```python
from build123d import *

# Parameters (mm, degrees)
F0_W      = 5.5
F0_H      = 9.5
F1_DEPTH  = 32
F2_SIZE   = 1
F3_R      = 1.5
F4_DEPTH  = 5.5
F5_W      = 1.5
F5_H      = 8
F6_DEPTH  = 9.5
F8_DEPTH  = 1
F10_DEPTH = 1
F11_R     = 1.5
F12_DEPTH = 9.5


with BuildPart() as f1:
    # F0 (on Top) → F1 (new body)
    with BuildSketch(Plane.XY):
        with Locations((2.75, 4.75)):
            Rectangle(F0_W, F0_H)
    extrude(amount=F1_DEPTH)

    # F2
    f2_edges = [f1.edges().sort_by_distance(p)[0] for p in [
        (2.75, 0, 32),
        (2.75, 9.5, 32),
    ]]
    chamfer(f2_edges, length=F2_SIZE)

    # F3 (on face) → F4 (cut, through all)
    with BuildSketch(Plane.YZ.offset(5.5)):
        with Locations((4.75, 3)):
            Circle(F3_R)
    extrude(amount=-F4_DEPTH, mode=Mode.SUBTRACT)

    # F5 (on face) → F6 (cut, through all)
    with BuildSketch(Plane(origin=(0, 9.5, 0), x_dir=(-1, 0, 0), z_dir=(0, 1, 0))):
        with Locations((-2.75, 4)):
            Rectangle(F5_W, F5_H)
    extrude(amount=-F6_DEPTH, mode=Mode.SUBTRACT)

    # F7 (on face) → F8 (cut)
    with BuildSketch(Plane.YZ.offset(5.5)):
        Polygon((9.5, 17), (0, 29), (0, 28), (9.5, 16), align=None)
    extrude(amount=-F8_DEPTH, mode=Mode.SUBTRACT)

    # F9 (on face) → F10 (cut)
    with BuildSketch(Plane(origin=(0, 0, 0), x_dir=(0, -1, 0), z_dir=(-1, 0, 0))):
        Polygon((0, 28), (0, 29), (-9.5, 17), (-9.5, 16), align=None)
    extrude(amount=-F10_DEPTH, mode=Mode.SUBTRACT)

    # F11 (on face) → F12 (cut, through all)
    with BuildSketch(Plane.XZ):
        with Locations((2.75, 21.25)):
            Circle(F11_R)
    extrude(amount=-F12_DEPTH, mode=Mode.SUBTRACT)


solid = f1.part
```
For this review, take the finished solid that the model builds, in its own axes (mm). A direction names the side the tool comes from. Round coordinates to 2 decimals unless told otherwise and drop trailing zeros. Write each loop counter-clockwise with the first axis right and the second up, starting at its lowest first coordinate (ties: lowest second). Pieces come first, ordered by that corner, then holes. Notation, with made-up numbers: (-25.5, -19) - (32.5, -19) arc R19 cw to (32.5, -5) - close; hole circle Ø9 at (10, 58.25). An arc over 180 degrees is marked (long way). Put each result on its own line as item: value.
Q1. Machinability: for faces 1 (the face through (4.5, 4.7, 22.5)), 2 (the face through (4.51, 5.44, 1.67)), 3 (the face through (2, 5, 5)), 4 (the face through (0.493, 4.684, 23.084)), which of the approach directions +Z, -Z, +X, -X, +Y, -Y give a long, thin tool a straight path to every point of the face, cutting with its end or side? Answer none if there is none.
Solved:
face 1: +X
face 2: +X, -X
face 3: -Z, +Y, -Y
face 4: -X
Q2. We need section D-D (x = 2.75). Give the boundary of the cut face in (y, z), and give its area (4 significant figures).
Solved:
outline: (0, 8) - (9.5, 8) - (9.5, 19.75) - (0, 19.75) - close; (0, 22.75) - (9.5, 22.75) - (9.5, 31) - (8.5, 32) - (1, 32) - (0, 31) - close
area: 198.5 mm2
Q3. We need section B-B (y = 4.75). Give the boundary of the cut face in (x, z), and give its area (3 significant figures).
Solved:
outline: (0, 0) - (2, 0) - (2, 1.5) - (0, 1.5) - close; (0, 4.5) - (2, 4.5) - (2, 8) - (3.5, 8) - (3.5, 4.5) - (5.5, 4.5) - (5.5, 22) - (4.5, 22) - (4.5, 23) - (5.5, 23) - (5.5, 32) - (0, 32) - (0, 23) - (1, 23) - (1, 22) - (0, 22) - close; (3.5, 0) - (5.5, 0) - (5.5, 1.5) - (3.5, 1.5) - close; hole circle Ø3 at (2.75, 21.25)
area: 143 mm2
Q4. We need section C-C (z = 6). Give the boundary of the cut face in (x, y), and give its area (3 significant figures).
Solved:
outline: (0, 0) - (2, 0) - (2, 9.5) - (0, 9.5) - close; (3.5, 0) - (5.5, 0) - (5.5, 9.5) - (3.5, 9.5) - close
area: 38.0 mm2
Q5. We need section A-A (x = 5.2). Give the boundary of the cut face in (y, z).
Solved:
outline: (0, 0) - (9.5, 0) - (9.5, 16) - (0, 28) - close; (0, 29) - (9.5, 17) - (9.5, 31) - (8.5, 32) - (1, 32) - (0, 31) - close; hole circle Ø3 at (4.75, 3)
Q6. Wall thickness on probe 1 along Z at (x, y) = (4.4, 4.75); probe 2 along Z at (x, y) = (0.8, 4.75); probe 3 along X at (y, z) = (4.5, 5.5): over which ranges is each line inside the solid? List them lowest first.
Solved:
probe 1: z = 0 to 1.5, 4.5 to 32
probe 2: z = 0 to 1.5, 4.5 to 22, 23 to 32
probe 3: x = 0 to 2, 3.5 to 5.5
Q7. Mouldability with a two-part tool opening along X and no side actions: class faces 5 (the face through (1, 4.8, 22.5)), 6 (the face through (5.007, 4.816, 22.916)), 7 (the face through (3.5, 5, 5)) as released by +X, released by -X, zero draft, split by the parting line, or undercut.
Solved:
face 5: released by -X
face 6: zero draft
face 7: undercut
